```python
from build123d import *

# Parameters (mm, degrees)
EXTRUDE_1_DEPTH     = 10
EXTRUDE_2_DEPTH     = 6
EXTRUDE_3_DEPTH     = 8
SKETCH_5_R          = 11
EXTRUDE_4_DEPTH     = 2
SKETCH_6_R          = 4.5
CUT_EXTRUDE_1_DEPTH = 3
SKETCH_7_R          = 2.5
EXTRUDE_5_DEPTH     = 25
CUT_EXTRUDE_START   = -22
CUT_EXTRUDE_2_DEPTH = 22
SKETCH_9_R          = 1.5
CUT_EXTRUDE_3_DEPTH = 10
SKETCH_10_W         = 17
SKETCH_10_H         = 10
EXTRUDE_6_DEPTH     = 5
SKETCH_11_W         = 14.973580244
SKETCH_11_H         = 4
CUT_EXTRUDE_4_DEPTH = 5
SKETCH_12_W         = 10
SKETCH_12_H         = 1.224563607
CUT_EXTRUDE_5_DEPTH = 5
SKETCH_13_W         = 0.8
SKETCH_13_H         = 0.8
EXTRUDE_7_DEPTH     = 5


with BuildPart() as part:
    # 草图1 → 凸台-拉伸1 (new body)
    with BuildSketch(Plane(origin=(0, 0, 0), x_dir=(1, 0, 0), z_dir=(0, 1, 0))):
        Polygon((-17, -21), (17, -21), (21, -17), (21, 17), (17, 21), (-17, 21), (-21, 17), (-21, -17), align=None)
    extrude(amount=EXTRUDE_1_DEPTH)

    # 草图3 → 凸台-拉伸2 (add)
    with BuildSketch(Plane(origin=(0, 10, 0), x_dir=(1, 0, 0), z_dir=(0, 1, 0))):
        Polygon((15, 21), (21, 15), (21, -15), (15, -21), (-15, -21), (-21, -15), (-21, 15), (-15, 21), align=None)
    extrude(amount=EXTRUDE_2_DEPTH)

    # 草图4 → 凸台-拉伸3 (add)
    with BuildSketch(Plane(origin=(0, 16, 0), x_dir=(1, 0, 0), z_dir=(0, 1, 0))):
        Polygon((15, 21), (-15, 21), (-17, 21), (-21, 17), (-21, 15), (-21, -15), (-21, -17), (-17, -21), (-15, -21), (15, -21), (17, -21), (21, -17), (21, -15), (21, 15), (21, 17), (17, 21), align=None)
    extrude(amount=EXTRUDE_3_DEPTH)

    # 草图5 → 凸台-拉伸4 (add)
    with BuildSketch(Plane(origin=(0, 24, 0), x_dir=(1, 0, 0), z_dir=(0, 1, 0))):
        with Locations(Location((0, 0, 0), (0, 0, 270))):
            Circle(SKETCH_5_R)
    extrude(amount=EXTRUDE_4_DEPTH)

    # 草图6 → 切除-拉伸1 (cut)
    with BuildSketch(Plane(origin=(0, 26, 0), x_dir=(1, 0, 0), z_dir=(0, 1, 0))):
        with Locations(Location((0, 0, 0), (0, 0, 270))):
            Circle(SKETCH_6_R)
    extrude(amount=-CUT_EXTRUDE_1_DEPTH, mode=Mode.SUBTRACT)

    # 草图7 → 凸台-拉伸5 (add)
    with BuildSketch(Plane(origin=(0, 23, 0), x_dir=(1, 0, 0), z_dir=(0, 1, 0))):
        with Locations(Location((0, 0, 0), (0, 0, 270))):
            Circle(SKETCH_7_R)
    extrude(amount=EXTRUDE_5_DEPTH)

    # 草图8 → 切除-拉伸2 (cut)
    with BuildSketch(Plane(origin=(0, 48, 0), x_dir=(1, 0, 0), z_dir=(0, 1, 0)).offset(CUT_EXTRUDE_START)):
        with BuildLine():
            Line((-1.5, 2), (1.5, 2))
            ThreePointArc((1.5, 2), (0, 2.5), (-1.5, 2))
        make_face()
    extrude(amount=CUT_EXTRUDE_2_DEPTH, mode=Mode.SUBTRACT)

    # 草图9 → 切除-拉伸3 (cut)
    with BuildSketch(Plane(origin=(0, 24, 0), x_dir=(1, 0, 0), z_dir=(0, 1, 0))):
        with Locations(Location((-15.5, 15.5, 0), (0, 0, 270))):
            Circle(SKETCH_9_R)
        with Locations(Location((15.5, 15.5, 0), (0, 0, 270))):
            Circle(SKETCH_9_R)
        with Locations(Location((15.5, -15.5, 0), (0, 0, 270))):
            Circle(SKETCH_9_R)
        with Locations(Location((-15.5, -15.5, 0), (0, 0, 270))):
            Circle(SKETCH_9_R)
    extrude(amount=-CUT_EXTRUDE_3_DEPTH, mode=Mode.SUBTRACT)

    # 草图10 → 凸台-拉伸6 (add)
    with BuildSketch(Plane.XY.offset(21)):
        with Locations((0, 5)):
            Rectangle(SKETCH_10_W, SKETCH_10_H)
    extrude(amount=EXTRUDE_6_DEPTH)

    # 草图11 → 切除-拉伸4 (cut)
    with BuildSketch(Plane.XY.offset(26)):
        with Locations((0, 7)):
            Rectangle(SKETCH_11_W, SKETCH_11_H)
    extrude(amount=-CUT_EXTRUDE_4_DEPTH, mode=Mode.SUBTRACT)

    # 草图12 → 切除-拉伸5 (cut)
    with BuildSketch(Plane.XY.offset(26)):
        with Locations((0, 9.612281804)):
            Rectangle(SKETCH_12_W, SKETCH_12_H)
    extrude(amount=-CUT_EXTRUDE_5_DEPTH, mode=Mode.SUBTRACT)

    # 草图13 → 凸台-拉伸7 (add)
    with BuildSketch(Plane.XY.offset(21)):
        with Locations((-5.5, 7)):
            Rectangle(SKETCH_13_W, SKETCH_13_H)
        with Locations((-3.3, 7)):
            Rectangle(SKETCH_13_W, SKETCH_13_H)
        with Locations((-1.1, 7)):
            Rectangle(SKETCH_13_W, SKETCH_13_H)
        with Locations((1.1, 7)):
            Rectangle(SKETCH_13_W, SKETCH_13_H)
        with Locations((3.3, 7)):
            Rectangle(SKETCH_13_W, SKETCH_13_H)
        with Locations((5.5, 7)):
            Rectangle(SKETCH_13_W, SKETCH_13_H)
    extrude(amount=EXTRUDE_7_DEPTH)


solid = part.part
```
Here's how the part is built. I have some questions about the finished solid (model axes, mm). A direction names the side the tool comes from. Give positions to 0.01 mm unless a question says otherwise; leave off trailing zeros. Loops run counter-clockwise (first coordinate to the right, second up) from the corner with the lowest first, then second, coordinate; pieces in that order, holes last. Notation, with made-up numbers: M 80.25,47.5 L 137.25,47.5 A28 ccw 137.25,66.5 Z; hole C 60,41 d9. An arc over 180 degrees is marked long. Use one line per item in the form item = value. Start each with the question number.
Q1. If we section it at C-C (y = 39): Write out the boundary of the cut face in (x, z).
Q2. If we section it at B-B (z = 18.5): Write out the boundary of the cut face in (x, y).
Q3. I need wall thicknesses on line 1 along X through (y, z) = (24.15, 0); line 2 along X through (y, z) = (18.5, 15.5); line 3 along Z through (x, y) = (15, 21). Which ranges of each line are inside material? Lowest first, please.
Q4. If we section it at A-A (x = 0): Write out the boundary of the cut face in (y, z).
Q5. If we section it at D-D (x = -12): Write out the boundary of the cut face in (y, z).
Q6. Thinking about a two-plate mould opening in Z: for faces 6 (the flat face through (-18.2, 16, -18.5)), 7 (the flat face through (18, 13, -18)), 8 (the flat face through (16, 14, -16)), 9 (the cylindrical face through (15.57, 19.07, 14)), which applies, +Z half, -Z half, draft (parallel to the pull), parting line (faces both ways), or undercut?
Q7. Which directions (+Z, -Z, +X, -X, +Y, -Y) give clear straight access to the entire face, cutting with the end or side of a thin tool? Please do faces 1 (the flat face through (0, 5, 24)), 2 (the flat face through (-18, 13, 18)), 3 (the flat face through (18, 13, 18)), 4 (the cylindrical face through (-15.43, 19.07, 14)), 5 (the flat face through (-18, 13, -18)).
Q8. Will these pins go through, and if not, where does the flat tip stop? pin 1 Ø8 at (x, z) = (-10, 17.5) entering from -Y; pin 2 Ø8 at (x, y) = (8.5, 25) entering from +Z; pin 3 Ø4 at (x, z) = (-3.5, 22.5) entering from +Y; pin 4 Ø0.9 at (y, z) = (7, 23) entering from +X.
Taken from the geometry:
q1.outline = M -1.5,-2 L 1.5,-2 A2.5 ccw long Z
q2.outline = M -19.5,0 L 19.5,0 L 19.5,10 L 17.5,10 L 17.5,16 L 19.5,16 L 19.5,24 L -19.5,24 L -19.5,16 L -17.5,16 L -17.5,10 L -19.5,10 Z
q3.line_1 = -11 to -4.5, -2.5 to 2.5, 4.5 to 11
q3.line_2 = -21 to -17, -14 to 14, 17 to 21
q3.line_3 = -21 to -16.91, -14.09 to 14.09, 16.91 to 21
q4.outline = M 0,-21 L 24,-21 L 24,-11 L 26,-11 L 26,-4.5 L 23,-4.5 L 23,-2.5 L 26,-2.5 L 26,-2 L 48,-2 L 48,2.5 L 23,2.5 L 23,4.5 L 26,4.5 L 26,11 L 24,11 L 24,21 L 5,21 L 5,26 L 0,26 Z
q5.outline = M 0,-21 L 24,-21 L 24,21 L 0,21 Z
q6.face_6 = draft
q6.face_7 = -Z half
q6.face_8 = undercut
q6.face_9 = undercut
q7.face_1 = +Z
q7.face_2 = +Z, -X
q7.face_3 = +Z, +X
q7.face_4 = +Y
q7.face_5 = -Z, -X
q8.pin_1 = 0
q8.pin_2 = 21
q8.pin_3 = 24
q8.pin_4 = 8.5
